Design review of the part built by this model. Coordinates are the model's own, in mm. Face numbers are marked on the shaded views. A direction names the side the tool comes from. Coordinates: 2 decimals unless noted, no trailing zeros. Loops run counter-clockwise (first coordinate to the right, second up) from the corner with the lowest first, then second, coordinate; pieces in that order, holes last. Notation, with made-up numbers: (-36.5, -24) -> (11.5, -24) arc R23 cw to (11.5, 15) -> close; hole circle Ø2 at (63.5, -17). An arc over 180 degrees is marked (long way). Use one line per item in the form item = value. Start each with the question number.
1. Consider section A-A (x = 0). State the section outline as (y, z) points, then the cut area to 3 significant figures.
2. Machinability: for the marked faces 5 and 6, which of the approach directions +Z, -Z, +X, -X, +Y, -Y give a long, thin tool a straight path to every point of the face, cutting with its end or side? Answer none if there is none.
3. Consider section D-D (x = 12.5). State the section outline as (y, z) points, then the cut area to 3 significant figures.
4. Consider section C-C (y = -62.5). State the section outline as (x, z) points.
5. Wall thickness on line 1 (Y direction, x = -22.7, z = -17.5); line 2 (X direction, y = -129, z = 3); line 3 (Y direction, x = 16.5, z = -12): over which ranges is each line inside the solid? List them lowest first. Write a range as from..to.
6. Consider section B-B (z = -17.5). State the section outline as (x, y) points, then the cut area to 3 significant figures.
7. The part is to be moulded in two halves that separate along Y. For the marked faces 1, 2, 3 and 4, say which applies: released by +Y, released by -Y, zero draft, split by the parting line, or undercut.
from build123d import *

# Parameters (mm, degrees)
SKETCH1_W           = 50
SKETCH1_H           = 50
BOSS_EXTRUDE1_DEPTH = 175
SHELL1_T            = -3
CUT_EXTRUDE1_REACH  = 177
SKETCH2_R           = 7.5
SKETCH2_R_2         = 2.15
SKETCH2_2_R         = 7.5
CUT_EXTRUDE2_DEPTH  = 176
SKETCH3_R           = 5
CUT_EXTRUDE3_DEPTH  = 51
FILLET1_R           = 1


with BuildPart() as part:
    # Sketch1 → Boss-Extrude1 (new body)
    with BuildSketch(Plane(origin=(0, 0, 0), x_dir=(1, 0, 0), z_dir=(0, 1, 0))):
        Rectangle(SKETCH1_W, SKETCH1_H)
    extrude(amount=-BOSS_EXTRUDE1_DEPTH)

    # Shell1
    shell1_openings = [part.faces().sort_by_distance(p)[0] for p in [
        (0, -87.5, -25),
        (0, -87.5, 25),
    ]]
    offset(amount=SHELL1_T, openings=shell1_openings, kind=Kind.INTERSECTION)

    # Sketch2 → Cut-Extrude1 (cut, up to next)
    with BuildSketch(Plane(origin=(0, 0, 0), x_dir=(1, 0, 0), z_dir=(0, 1, 0)), mode=Mode.PRIVATE) as cut_extrude1_sk1:
        Circle(SKETCH2_R)
    cut_extrude1_tool1 = extrude(cut_extrude1_sk1.sketch, amount=-CUT_EXTRUDE1_REACH, mode=Mode.PRIVATE) & part.part
    add(cut_extrude1_tool1.solids().sort_by_distance((0, 0, 0))[0], mode=Mode.SUBTRACT)
    # Sketch2 → Cut-Extrude1 (cut, up to next)
    with BuildSketch(Plane(origin=(0, 0, 0), x_dir=(1, 0, 0), z_dir=(0, 1, 0)), mode=Mode.PRIVATE) as cut_extrude1_sk2:
        with Locations((-12.5, 0)):
            Circle(SKETCH2_R_2)
    cut_extrude1_tool2 = extrude(cut_extrude1_sk2.sketch, amount=-CUT_EXTRUDE1_REACH, mode=Mode.PRIVATE) & part.part
    add(cut_extrude1_tool2.solids().sort_by_distance((-12.5, 0, 0))[0], mode=Mode.SUBTRACT)
    # Sketch2 → Cut-Extrude1 (cut, up to next)
    with BuildSketch(Plane(origin=(0, 0, 0), x_dir=(1, 0, 0), z_dir=(0, 1, 0)), mode=Mode.PRIVATE) as cut_extrude1_sk3:
        with Locations((12.5, 0)):
            Circle(SKETCH2_R_2)
    cut_extrude1_tool3 = extrude(cut_extrude1_sk3.sketch, amount=-CUT_EXTRUDE1_REACH, mode=Mode.PRIVATE) & part.part
    add(cut_extrude1_tool3.solids().sort_by_distance((12.5, 0, 0))[0], mode=Mode.SUBTRACT)

    # Sketch2_2 → Cut-Extrude2 (cut, through all)
    with BuildSketch(Plane(origin=(0, 0, 0), x_dir=(1, 0, 0), z_dir=(0, 1, 0))):
        Circle(SKETCH2_2_R)
    extrude(amount=-CUT_EXTRUDE2_DEPTH, mode=Mode.SUBTRACT)

    # Sketch3 → Cut-Extrude3 (cut, through all)
    with BuildSketch(Plane(origin=(25, 0, 0), x_dir=(0, 0, -1), z_dir=(1, 0, 0))):
        with Locations((17.5, -20)):
            Circle(SKETCH3_R)
        with Locations((17.5, -80)):
            Circle(SKETCH3_R)
    extrude(amount=-CUT_EXTRUDE3_DEPTH, mode=Mode.SUBTRACT)

    # Fillet1
    fillet1_edges = [part.edges().sort_by_distance(p)[0] for p in [
        (25, -175, 0),
        (0, -175, -25),
        (-25, -175, 0),
        (0, 0, -25),
        (25, 0, 0),
        (0, 0, 25),
        (-25, 0, 0),
        (-25, -87.5, -25),
        (25, -87.5, -25),
        (25, -87.5, 25),
        (-25, -87.5, 25),
        (0, -175, 25),
    ]]
    fillet(fillet1_edges, radius=FILLET1_R)


solid = part.part
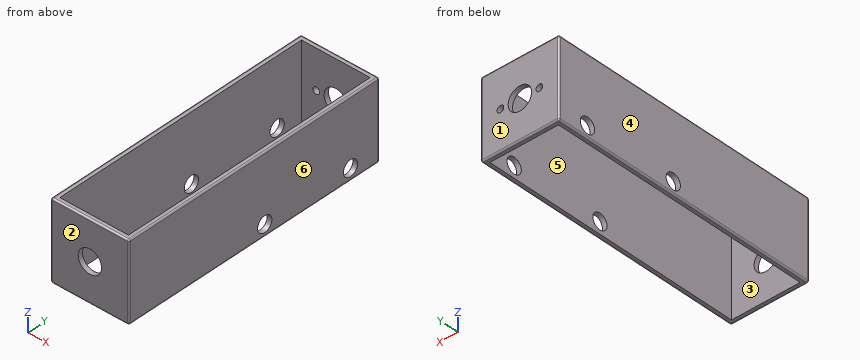
Geometry check:
q1.outline = (-175, -24) arc R1 ccw to (-174, -25) -> (-172, -25) -> (-172, -7.5) -> (-175, -7.5) -> close; (-175, 7.5) -> (-172, 7.5) -> (-172, 25) -> (-174, 25) arc R1 ccw to (-175, 24) -> close; (-3, -25) -> (-1, -25) arc R1 ccw to (0, -24) -> (0, -7.5) -> (-3, -7.5) -> close; (-3, 7.5) -> (0, 7.5) -> (0, 24) arc R1 ccw to (-1, 25) -> (-3, 25) -> close
q1.area = 209 mm²
q2.face_5 = +Z, -Z
q2.face_6 = +Z, -Z, +X, +Y, -Y
q3.outline = (-175, -24) arc R1 ccw to (-174, -25) -> (-172, -25) -> (-172, 25) -> (-174, 25) arc R1 ccw to (-175, 24) -> close; (-3, -25) -> (-1, -25) arc R1 ccw to (0, -24) -> (0, -2.15) -> (-3, -2.15) -> close; (-3, 2.15) -> (0, 2.15) -> (0, 24) arc R1 ccw to (-1, 25) -> (-3, 25) -> close
q3.area = 286 mm²
q4.outline = (-25, -24) arc R1 ccw to (-24, -25) -> (-22, -25) -> (-22, 25) -> (-24, 25) arc R1 ccw to (-25, 24) -> close; (22, -25) -> (24, -25) arc R1 ccw to (25, -24) -> (25, 24) arc R1 ccw to (24, 25) -> (22, 25) -> close
q5.line_1 = -175..-85, -75..-25, -15..0
q5.line_2 = -25..-22, 22..25
q5.line_3 = -175..-172, -3..0
q6.outline = (-25, -174) arc R1 ccw to (-24, -175) -> (24, -175) arc R1 ccw to (25, -174) -> (25, -85) -> (22, -85) -> (22, -172) -> (-22, -172) -> (-22, -85) -> (-25, -85) -> close; (-25, -75) -> (-22, -75) -> (-22, -25) -> (-25, -25) -> close; (-25, -15) -> (-22, -15) -> (-22, -3) -> (22, -3) -> (22, -15) -> (25, -15) -> (25, -1) arc R1 ccw to (24, 0) -> (-24, 0) arc R1 ccw to (-25, -1) -> close; (22, -75) -> (25, -75) -> (25, -25) -> (22, -25) -> close
q6.area = 1,190 mm²
q7.face_1 = released by +Y
q7.face_2 = released by -Y
q7.face_3 = undercut
q7.face_4 = zero draft
